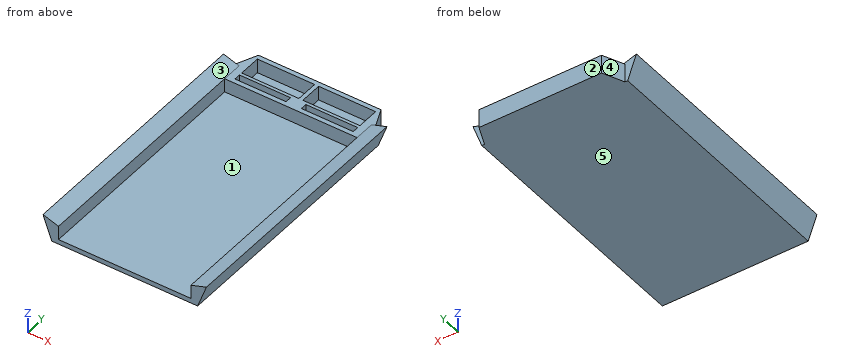
```python
from build123d import *

# Parameters (mm, degrees)
F1_DEPTH = 127
F3_DEPTH = 10.16
F4_W     = 65.889194
F4_H     = 6.89044
F5_DEPTH = 10.16
F7_DEPTH = 25.4
F8_W     = 25.775215
F8_H     = 3.177766
F8_W_2   = 25.416197
F9_DEPTH = 7.112


with BuildPart() as f1:
    # F0 (on Front) → F1 (new body)
    with BuildSketch(Plane.XZ):
        Polygon((-40.653061, 5.938083), (-36.282156, -5.938083), (36.282156, -5.938083), (40.653061, 5.938083), (32.944597, 3.345205), (32.944597, -3.545235), (0, -3.545235), (-32.944597, -3.545235), (-32.944597, 3.345205), align=None)
    extrude(amount=F1_DEPTH)

    # F2 (on face) → F3 (join)
    with BuildSketch(Plane(origin=(0, 0, 0), x_dir=(-1, 0, 0), z_dir=(0, 1, 0))):
        Polygon((-34.912035, 3.345205), (-34.912035, -5.938083), (34.912035, -5.938083), (34.912035, 3.345205), (-32.944597, 3.345205), align=None)
    extrude(amount=F3_DEPTH)

    # F4 (on face) → F5 (join)
    with BuildSketch(Plane.XZ):
        with Locations((0, -0.100015)):
            Rectangle(F4_W, F4_H)
    extrude(amount=F5_DEPTH)

    # F6 (on face) → F7 (cut)
    with BuildSketch(Plane.XY.offset(3.345205)):
        Polygon((30.480051, 10.16), (34.912035, 0), (34.912035, 10.16), align=None)
        Polygon((-34.912035, 10.16), (-34.912035, 0), (-30.480051, 10.16), align=None)
    extrude(amount=-F7_DEPTH, mode=Mode.SUBTRACT)

    # F8 (on face) → F9 (cut)
    with BuildSketch(Plane.XY.offset(3.345205)):
        with Locations((16.533188, -6.29418)):
            Rectangle(F8_W, F8_H)
        Polygon((29.420795, -3.175261), (29.420795, 7.883063), (1.056288, 7.883063), (1.056288, -3.175261), (3.64558, -3.175261), align=None)
        with Locations((-16.712696, -6.29418)):
            Rectangle(F8_W_2, F8_H)
        Polygon((-29.420795, 7.883063), (-29.420795, -3.175261), (-4.004598, -3.175261), (-0.944527, -3.175261), (-0.944527, 7.883063), align=None)
    extrude(amount=-F9_DEPTH, mode=Mode.SUBTRACT)


solid = f1.part
```
Design review of the part built by this model. Coordinates are the model's own, in mm. Face numbers are marked on the shaded views. A direction names the side the tool comes from. Coordinates: 2 decimals unless noted, no trailing zeros. Loops run counter-clockwise (first coordinate to the right, second up) from the corner with the lowest first, then second, coordinate; pieces in that order, holes last. Notation, with made-up numbers: (12.5, 85.5) -> (23.5, 85.5) arc R14 ccw to (23.5, 106.5) -> close; hole circle Ø4 at (-2, -35.5). An arc over 180 degrees is marked (long way). Answer as a JSON object with one key per item and string values.
Q1. Take a section at B-B on y = -56.5. Give the boundary of the cut face in (x, z), plus the area to 3 significant figures.
Answer block:
{"outline": "(-40.65, 5.94) -> (-36.28, -5.94) -> (36.28, -5.94) -> (40.65, 5.94) -> (32.94, 3.35) -> (32.94, -3.55) -> (-32.94, -3.55) -> (-32.94, 3.35) -> close", "area": "269 mm^2"}
Q2. Clearance check with flat-ended pins moving along their axes: pin 1 Ø1.5 at (y, z) = (-42.5, 3) entering from +X; pin 2 Ø12 at (x, y) = (-7, -49.5) entering from +Z; pin 3 Ø2.5 at (y, z) = (-7, -1) entering from +X. State where each tip first meets the part, or that it passes through.
Answer block:
{"pin 1": "stops at x = 39.85", "pin 2": "stops at z = -3.55", "pin 3": "stops at x = 38.56"}
Q3. Tool access review of the marked faces 1 and 2: name each direction out of +Z, -Z, +X, -X, +Y, -Y from which nothing blocks a thin tool from reaching the whole face with its end or side.
Answer block:
{"face 1": "+Z, -Y", "face 2": "+Z, -Z, +X, -X, +Y"}
Q4. Take a section at C-C on x = -15.5. Give the boundary of the cut face in (y, z), plus the area to 3 significant figures.
Answer block:
{"outline": "(-127, -5.94) -> (10.16, -5.94) -> (10.16, 3.35) -> (7.88, 3.35) -> (7.88, -3.77) -> (-3.18, -3.77) -> (-3.18, 3.35) -> (-4.71, 3.35) -> (-4.71, -3.77) -> (-7.88, -3.77) -> (-7.88, 3.35) -> (-10.16, 3.35) -> (-10.16, -3.55) -> (-127, -3.55) -> close", "area": "367 mm^2"}
Q5. Take a section at A-A on z = -2.25. Give the boundary of the cut face in (x, y).
Answer block:
{"outline": "(-37.64, -127) -> (-32.94, -127) -> (-32.94, -10.16) -> (32.94, -10.16) -> (32.94, -127) -> (37.64, -127) -> (37.64, 0) -> (34.91, 0) -> (30.48, 10.16) -> (-30.48, 10.16) -> (-34.91, 0) -> (-37.64, 0) -> close; hole (-29.42, -7.88) -> (-4, -7.88) -> (-4, -4.71) -> (-29.42, -4.71) -> close; hole (-29.42, -3.18) -> (-0.94, -3.18) -> (-0.94, 7.88) -> (-29.42, 7.88) -> close; hole (1.06, -3.18) -> (29.42, -3.18) -> (29.42, 7.88) -> (1.06, 7.88) -> close; hole (3.65, -7.88) -> (29.42, -7.88) -> (29.42, -4.71) -> (3.65, -4.71) -> close"}
Q6. The part is to be moulded in two halves that separate along X. For the marked faces 3, 4 and 5, say which applies: +X half, -X half, draft (parallel to the pull), parting line (faces both ways), or undercut.
Answer block:
{"face 3": "undercut", "face 4": "-X half", "face 5": "draft"}
Q7. To check wall thickness, follow L1, parallel to Y at x = -18, z = -1.25; L2, parallel to Z at x = 11, y = -40; L3, parallel to Z at x = -16, y = -8.5. State the ranges of each line that lie inside material, in increasing order.
Answer block:
{"L1": "y = -10.16 to -7.88, -4.71 to -3.18, 7.88 to 10.16", "L2": "z = -5.94 to -3.55", "L3": "z = -5.94 to 3.35"}
